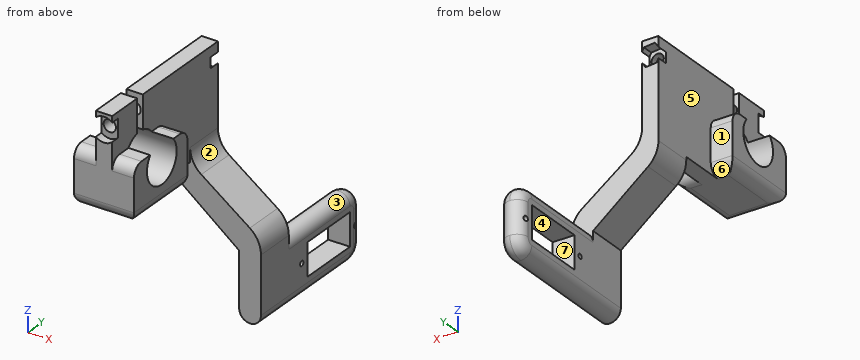
from build123d import *

# Parameters (mm, degrees)
SKETCH1_R                                        = 0.9
SKETCH1_W                                        = 12
SKETCH1_H                                        = 23
BOSS_EXTRUDE1_DEPTH                              = 32
CBORE_FOR_M4_PAN_HEAD_MACHINE_SCREW2_D           = 4.5
CBORE_FOR_M4_PAN_HEAD_MACHINE_SCREW2_CBORE_D     = 9
CBORE_FOR_M4_PAN_HEAD_MACHINE_SCREW2_CBORE_DEPTH = 3.1
CUT_EXTRUDE2_DEPTH                               = 4
SKETCH9_W                                        = 35
SKETCH9_H                                        = 57
CUT_EXTRUDE3_DEPTH                               = 26
SKETCH10_W                                       = 24
SKETCH10_H                                       = 54
CUT_EXTRUDE4_DEPTH                               = 24
BOSS_EXTRUDE2_DEPTH                              = 8
BOSS_EXTRUDE2_DEPTH_BACK                         = 14
FILLET3_R                                        = 4
FILLET4_R                                        = 6
FILLET5_R                                        = 4
CUT_EXTRUDE5_DEPTH                               = 86.654277555
FILLET6_R                                        = 10


with BuildPart() as part:
    # Sketch1 → Boss-Extrude1 (new body)
    with BuildSketch(Plane(origin=(0, 0, 0), x_dir=(0, 0, -1), z_dir=(1, 0, 0))):
        with BuildLine():
            Line((-55.350295908, -42.411439664), (-43.208412731, -42.411439664))
            ThreePointArc((-43.208412731, -42.411439664), (-27.350295908, -43.911439664), (-43.208412731, -45.411439664))
            Line((-43.208412731, -45.411439664), (-55.350295908, -45.411439664))
            Line((-55.350295908, -45.411439664), (-55.350295908, -58.911439664))
            Line((-55.350295908, -58.911439664), (-20.350295908, -58.911439664))
            Line((-20.350295908, -58.911439664), (-20.350295908, -16.911439664))
            Line((-20.350295908, -16.911439664), (28.649704092, -16.911439664))
            Line((28.649704092, -16.911439664), (28.649704092, 37.088560336))
            Line((28.649704092, 37.088560336), (4.649704092, 37.088560336))
            Line((4.649704092, 37.088560336), (4.649704092, -1.911439664))
            Line((4.649704092, -1.911439664), (-55.350295908, -1.911439664))
            Line((-55.350295908, -1.911439664), (-55.350295908, -28.911439664))
            Line((-55.350295908, -28.911439664), (-55.350295908, -42.411439664))
        make_face()
        with Locations((16.649704092, 34.088560336)):
            Circle(SKETCH1_R, mode=Mode.SUBTRACT)
        with Locations((16.649704092, 5.088560336)):
            Circle(SKETCH1_R, mode=Mode.SUBTRACT)
        with Locations((16.649704092, 19.588560336)):
            Rectangle(SKETCH1_W, SKETCH1_H, mode=Mode.SUBTRACT)
    extrude(amount=BOSS_EXTRUDE1_DEPTH)

    # CBORE for M4 Pan Head Machine Screw2 (through all)
    with Locations(Plane(origin=(0, -58.911439664, 0), x_dir=(-1, 0, 0), z_dir=(0, -1, 0))):
        with Locations((-3, -49.720295908)):
            CounterBoreHole(CBORE_FOR_M4_PAN_HEAD_MACHINE_SCREW2_D / 2, CBORE_FOR_M4_PAN_HEAD_MACHINE_SCREW2_CBORE_D / 2, CBORE_FOR_M4_PAN_HEAD_MACHINE_SCREW2_CBORE_DEPTH)

    # Sketch7 → Cut-Extrude2 (cut)
    with BuildSketch(Plane(origin=(0, -1.911439664, 0), x_dir=(1, 0, 0), z_dir=(0, 1, 0))):
        Polygon((7.082253493, -49.348086624), (4.718784051, -45.998856036), (0.636530558, -46.37106532), (-1.082253493, -50.092505192), (1.281215949, -53.441735779), (5.363469442, -53.069526496), align=None)
    extrude(amount=-CUT_EXTRUDE2_DEPTH, mode=Mode.SUBTRACT)

    # Sketch9 → Cut-Extrude3 (cut)
    with BuildSketch(Plane(origin=(32, 0, 0), x_dir=(0, 0, -1), z_dir=(1, 0, 0))):
        with Locations((-37.850295908, -30.411439664)):
            Rectangle(SKETCH9_W, SKETCH9_H)
    extrude(amount=-CUT_EXTRUDE3_DEPTH, mode=Mode.SUBTRACT)

    # Sketch10 → Cut-Extrude4 (cut)
    with BuildSketch(Plane.ZY):
        with Locations((-16.649704092, 10.088560336)):
            Rectangle(SKETCH10_W, SKETCH10_H)
    extrude(amount=-CUT_EXTRUDE4_DEPTH, mode=Mode.SUBTRACT)

    # Sketch11 → Boss-Extrude2 (add, two sides: drawn at the far end of the back side and taken through both)
    with BuildSketch(Plane.ZY.offset(-BOSS_EXTRUDE2_DEPTH_BACK)):
        with BuildLine():
            Line((20.350295908, -30.109144798), (40.350295908, -30.109144798))
            Line((40.350295908, -30.109144798), (40.350295908, -37.666441665))
            ThreePointArc((40.350295908, -37.666441665), (27.350295908, -43.911439664), (40.350295908, -50.156437662))
            Line((40.350295908, -50.156437662), (40.350295908, -58.911439664))
            Line((40.350295908, -58.911439664), (20.350295908, -58.911439664))
            Line((20.350295908, -58.911439664), (20.350295908, -30.109144798))
        make_face()
    extrude(amount=BOSS_EXTRUDE2_DEPTH + BOSS_EXTRUDE2_DEPTH_BACK)

    # Fillet3
    fillet3_edges = [part.edges().sort_by_distance(p)[0] for p in [
        (3, -58.911439664, 20.350295908),
        (14, -44.510292231, 20.350295908),
        (-4, -30.109144798, 20.350295908),
        (10, -30.109144798, 20.350295908),
        (-4, -30.109144798, 40.350295908),
        (10, -30.109144798, 40.350295908),
        (-4, -58.911439664, 40.350295908),
        (10, -58.911439664, 40.350295908),
        (-8, -44.510292231, 20.350295908),
    ]]
    fillet(fillet3_edges, radius=FILLET3_R)

    # Fillet4
    fillet4_edges = [part.edges().sort_by_distance(p)[0] for p in [
        (28, 37.088560336, -4.649704092),
        (28, 37.088560336, -28.649704092),
    ]]
    fillet(fillet4_edges, radius=FILLET4_R)

    # Fillet5
    # the kernel refuses this fillet: 4 mm, written as the material it takes off along each edge
    with BuildSketch(Plane(origin=(32, 31.088560336, -4.649704092), x_dir=(-1, 0, 0), z_dir=(0, -1, 0)), Plane(origin=(24, -1.911439664, -4.649704092), x_dir=(1, 0, 0), z_dir=(0, 1, 0))) as fillet5_piece_1:
        with BuildLine():
            CenterArc((FILLET5_R, FILLET5_R), FILLET5_R, 180, 90)
            Line((0, FILLET5_R), (0, 0))
            Line((0, 0), (FILLET5_R, 0))
        make_face()
    extrude(amount=33, mode=Mode.SUBTRACT)
    with BuildSketch(Plane(origin=(32, 31.088560336, -10.649704092), x_dir=(0, 0, 1), z_dir=(0, -1, 0))) as fillet5_piece_2:
        with BuildLine():
            CenterArc((6 - FILLET5_R, FILLET5_R), FILLET5_R, 270, 90)
            Line((6 - FILLET5_R, 0), (6, 0))
            Line((6, 0), (6, FILLET5_R))
        make_face()
    revolve(axis=Axis((32, 31.088560336, -10.649704092), (-1, 0, 0)), revolution_arc=90, mode=Mode.SUBTRACT)
    with BuildSketch(Plane(origin=(32, 37.088560336, -22.649704092), x_dir=(0, -1, 0), z_dir=(0, 0, 1)), Plane(origin=(24, 37.088560336, -10.649704092), x_dir=(0, -1, 0), z_dir=(0, 0, -1))) as fillet5_piece_3:
        with BuildLine():
            CenterArc((FILLET5_R, -FILLET5_R), FILLET5_R, 90, 90)
            Line((0, -FILLET5_R), (0, 0))
            Line((0, 0), (FILLET5_R, 0))
        make_face()
    extrude(amount=12, mode=Mode.SUBTRACT)
    with BuildSketch(Plane(origin=(32, 31.088560336, -22.649704092), x_dir=(0, 1, 0), z_dir=(0, 0, 1))) as fillet5_piece_4:
        with BuildLine():
            CenterArc((6 - FILLET5_R, FILLET5_R), FILLET5_R, 270, 90)
            Line((6, FILLET5_R), (6, 0))
            Line((6, 0), (6 - FILLET5_R, 0))
        make_face()
    revolve(axis=Axis((32, 31.088560336, -22.649704092), (-1, 0, 0)), revolution_arc=90, mode=Mode.SUBTRACT)
    with BuildSketch(Plane(origin=(24, 31.088560336, -10.649704092), x_dir=(0, 0, 1), z_dir=(0, -1, 0))) as fillet5_piece_5:
        with BuildLine():
            CenterArc((6 - FILLET5_R, -FILLET5_R), FILLET5_R, 0, 90)
            Line((6, -FILLET5_R), (6, 0))
            Line((6, 0), (6 - FILLET5_R, 0))
        make_face()
    revolve(axis=Axis((24, 31.088560336, -10.649704092), (-1, 0, 0)), revolution_arc=90, mode=Mode.SUBTRACT)
    with BuildSketch(Plane(origin=(24, 31.088560336, -22.649704092), x_dir=(0, 1, 0), z_dir=(0, 0, 1))) as fillet5_piece_6:
        with BuildLine():
            CenterArc((6 - FILLET5_R, -FILLET5_R), FILLET5_R, 0, 90)
            Line((6, -FILLET5_R), (6, 0))
            Line((6, 0), (6 - FILLET5_R, 0))
        make_face()
    revolve(axis=Axis((24, 31.088560336, -22.649704092), (-1, 0, 0)), revolution_arc=90, mode=Mode.SUBTRACT)
    with BuildSketch(Plane(origin=(32, -26.911439664, -28.649704092), x_dir=(0, 0, 1), z_dir=(0, 1, 0)), Plane(origin=(24, 31.088560336, -28.649704092), x_dir=(0, 0, 1), z_dir=(0, -1, 0))) as fillet5_piece_7:
        with BuildLine():
            CenterArc((FILLET5_R, -FILLET5_R), FILLET5_R, 90, 90)
            Line((0, -FILLET5_R), (0, 0))
            Line((0, 0), (FILLET5_R, 0))
        make_face()
    extrude(amount=58, mode=Mode.SUBTRACT)

    # Sketch13 → Cut-Extrude5 (cut, through all)
    with BuildSketch(Plane(origin=(0, -1.911439664, 0), x_dir=(1, 0, 0), z_dir=(0, 1, 0))):
        Polygon((6, -20.350295908), (32, -1.350295908), (32, -20.350295908), align=None)
        Polygon((0, 4.649704092), (24, 4.649704092), (0, -14.350295908), align=None)
    extrude(amount=-CUT_EXTRUDE5_DEPTH, mode=Mode.SUBTRACT)

    # Fillet6
    fillet6_edges = [part.edges().sort_by_distance(p)[0] for p in [
        (6, -9.411439664, 20.350295908),
        (32, -9.411439664, 1.350295908),
        (0, -9.411439664, 14.350295908),
    ]]
    fillet(fillet6_edges, radius=FILLET6_R)


solid = part.part
Here's how the part is built. I have some questions about the finished solid (model axes, mm). Face numbers are marked on the shaded views. A direction names the side the tool comes from. Coordinates: 2 decimals unless noted, no trailing zeros. Write each loop counter-clockwise with the first axis right and the second up, starting at its lowest first coordinate (ties: lowest second). Pieces come first, ordered by that corner, then holes.
Item 1: On a 3-axis mill with a long thin cutter (end or side, diameter ignored), from which of +Z, -Z, +X, -X, +Y, -Y can I reach the whole of each face in a straight line? I mean the marked faces 1, 2, 3 and 4. Say none if no direction works.
Item 2: If I drill on line 1 (Z direction, x = 3, y = -49); line 2 (Z direction, x = 3, y = -20); line 3 (X direction, y = -11, z = 45), over which ranges is the centre line in solid material (lowest first)?
Item 3: I want a section at A-A on y = 17. Write out the boundary of the cut face in (x, z).
Item 4: I want a section at B-B on x = 26. Count the separate pieces of the cut face and the enclosed holes in it, and give its area (3 significant figures).
Item 5: Will these pins go through, and if not, where does the flat tip stop? pin 1 (9 mm diameter, centred on x = 28, z = -16.5, fed in from -Y); pin 2 (5 mm diameter, centred on x = 3.5, z = 50.5, fed in from +Y); pin 3 (11 mm diameter, centred on y = -51, z = 49.5, fed in from -X).
Item 6: If we mould it in two halves opening along Z, with no side actions, what happens to the marked faces 5, 6 and 7? For each: +Z half, -Z half, draft (parallel to the pull), parting line (faces both ways), or undercut.
Item 7: I want a section at C-C on x = 18. Write out the boundary of the cut face in (y, z).
Findings below:
1. face 1: +Z, -Z, -X, +Y
1. face 2: +Z, +X, +Y
1. face 3: +Z, +Y
1. face 4: +X, -X
2. line 1: z = 20.35 to 29.18, 41.52 to 47.47, 51.97 to 55.35
2. line 2: z = 20.35 to 47.47, 51.97 to 55.35
2. line 3: x = 0 to 6
3. outline: (24, -24.65) arc R4 ccw to (32, -24.65) - (32, -22.65) - (24, -22.65) - close; (24, -10.65) - (32, -10.65) - (32, -8.65) arc R4 ccw to (24, -8.65) - close
4. separate pieces: 1
4. enclosed holes: 3
4. area: 1,100 mm2
5. pin 1: stops at y = -16.91
5. pin 2: stops at y = -5.91
5. pin 3: stops at x = 0
6. face 5: draft
6. face 6: -Z half
6. face 7: undercut
7. outline: (-16.91, 0.1) - (-1.91, 0.1) - (-1.91, 11.58) - (-16.91, 11.58) - close
